Work out the finished part from the listing and answer in its coordinate system (mm). A direction names the side the tool comes from. Round coordinates to 2 decimals unless told otherwise and drop trailing zeros. Write each loop counter-clockwise with the first axis right and the second up, starting at its lowest first coordinate (ties: lowest second). Pieces come first, ordered by that corner, then holes.
1. Straight lines are drawn through the part: probe 1 along Y at (x, z) = (62, 16.5); probe 2 along X at (y, z) = (16, 38). For each, find the intervals that lie inside material, in ascending order.
2. Find section B-B (x = 43). Write down the section's boundary in (y, z).
3. Flat-ended cylindrical pins translate along their axes: pin 1 Ø16.5 at (y, z) = (100.94, 32.6) entering from +X; pin 2 Ø1 at (y, z) = (52, 75.5) entering from -X; pin 3 Ø10 at (y, z) = (30.5, 144.5) entering from +X. Find the tip coordinate at first contact, or state that the pin passes through.
4. Find section A-A (z = 125.5). Write down the section's boundary in (x, y), and give its area (3 significant figures).
5. Determine the mould class of faces 3 (the face through (14, 44, 0)), 4 (the face through (-2.348, 94.743, 33.981)), 5 (the face through (16.27, 41.85, 81.39)) for opening direction Z: pulls with the +Z half, pulls with the -Z half, needs draft (parallel to the pull), parting line crosses it, or undercut.
6. A tool of negligible diameter and unlimited length cuts with its end or side. For faces 1 (the face through (-2.35, 95.31, 131.27)), 2 (the face through (52, 0, 81)), from which of +Z, -Z, +X, -X, +Y, -Y can it reach the whole face along a straight path? Write none if from no direction.
```python
from build123d import *

# Parameters (mm, degrees)
EXTRUDE_THIN1_DEPTH = 165.1
SKETCH2_R           = 6.35
CUT_EXTRUDE1_DEPTH  = 5.7625


with BuildPart() as part:
    # Sketch1 → Extrude-Thin1 (new body)
    with BuildSketch(Plane.XY):
        Polygon((0, 120.65), (0, 82.55), (32.995567884, 0), (71.095567884, 0), (71.095567884, -4.7625), (29.770312185, -4.7625), (-4.7625, 81.633456448), (-4.7625, 120.65), align=None)
    extrude(amount=EXTRUDE_THIN1_DEPTH)

    # Sketch2 → Cut-Extrude1 (cut, through all)
    with BuildSketch(Plane(origin=(0, 0, 0), x_dir=(0, 0, -1), z_dir=(1, 0, 0))):
        with Locations((-134.204880657, 100.94227704)):
            Circle(SKETCH2_R)
        with Locations((-32.604880657, 100.94227704)):
            Circle(SKETCH2_R)
    extrude(amount=-CUT_EXTRUDE1_DEPTH, mode=Mode.SUBTRACT)


solid = part.part
```
Worked answers:
1. probe 1: y = -4.76 to 0
1. probe 2: x = 21.47 to 26.6
2. outline: (-4.76, 0) - (0, 0) - (0, 165.1) - (-4.76, 165.1) - close
3. pin 1: stops at x = 0
3. pin 2: stops at x = 6.88
3. pin 3: stops at x = 22.8
4. outline: (-4.76, 81.63) - (29.77, -4.76) - (71.1, -4.76) - (71.1, 0) - (33, 0) - (0, 82.55) - (0, 120.65) - (-4.76, 120.65) - close
4. area: 806 mm2
5. face 3: pulls with the -Z half
5. face 4: undercut
5. face 5: needs draft
6. face 1: +X, -X
6. face 2: +Z, -Z, +X, +Y
